```python
from build123d import *

# Parameters (mm, degrees)
F0_W     = 127
F0_H     = 127
F1_DEPTH = 127
F2_R     = 25.4
F3_R     = 12.7
F4_DEPTH = 50
F5_R     = 5
F6_DEPTH = 47
F7_R     = 5


# Not quite as in the source:
# - two fillets or chamfers of one size are made in one step


with BuildPart() as f1:
    # F0 (on Front) → F1 (new body)
    with BuildSketch(Plane.XZ):
        Rectangle(F0_W, F0_H)
    extrude(amount=F1_DEPTH)

    # F2
    f2_edges = [f1.edges().sort_by_distance(p)[0] for p in [
        (-63.5, -127, 0),
        (63.5, -127, 0),
        (-63.5, 0, 0),
        (63.5, 0, 0),
    ]]
    fillet(f2_edges, radius=F2_R)

    # F3
    f3_edges = [f1.edges().sort_by_distance(p)[0] for p in [
        (-63.5, -63.5, 63.5),
        (0, -127, -63.5),
        (63.5, -63.5, -63.5),
        (56.060512, -7.439488, -63.5),
        (56.060512, -119.560512, -63.5),
        (0, 0, -63.5),
        (-56.060512, -7.439488, -63.5),
        (-56.060512, -119.560512, -63.5),
        (-63.5, -63.5, -63.5),
    ]]
    fillet(f3_edges, radius=F3_R)

    # F4 (add): a face of the model
    f4_faces = [f1.faces().sort_by_distance(p)[0] for p in [
        (0, -63.5, 63.5),
    ]]
    extrude(f4_faces, amount=F4_DEPTH)

    # F5
    f5_edges = [f1.edges().sort_by_distance(p)[0] for p in [
        (-50.8, -63.5, 63.5),
        (-47.080256, -16.419744, 63.5),
        (-50.8, -63.5, 113.5),
        (-47.080256, -110.580256, 63.5),
        (0, -12.7, 63.5),
        (-47.080256, -16.419744, 113.5),
        (-47.080256, -110.580256, 113.5),
        (0, -12.7, 113.5),
        (0, -114.3, 113.5),
        (47.080256, -16.419744, 113.5),
        (47.080256, -110.580256, 113.5),
        (50.8, -63.5, 113.5),
        (0, -114.3, 63.5),
        (47.080256, -16.419744, 63.5),
        (47.080256, -110.580256, 63.5),
        (50.8, -63.5, 63.5),
    ]]
    fillet(f5_edges, radius=F5_R)

    # F6 (add): a face of the model
    f6_faces = [f1.faces().sort_by_distance(p)[0] for p in [
        (0, -63.5, 113.5),
    ]]
    extrude(f6_faces, amount=F6_DEPTH)

    # F7
    f7_edges = [f1.edges().sort_by_distance(p)[0] for p in [
        (-45.8, -63.5, 113.5),
        (-43.544722, -19.955278, 113.5),
        (-45.8, -63.5, 160.5),
        (-43.544722, -107.044722, 113.5),
        (0, -17.7, 113.5),
        (-43.544722, -19.955278, 160.5),
        (-43.544722, -107.044722, 160.5),
        (0, -17.7, 160.5),
        (0, -109.3, 160.5),
        (43.544722, -19.955278, 160.5),
        (43.544722, -107.044722, 160.5),
        (45.8, -63.5, 160.5),
        (0, -109.3, 113.5),
        (43.544722, -19.955278, 113.5),
        (43.544722, -107.044722, 113.5),
        (45.8, -63.5, 113.5),
    ]]
    fillet(f7_edges, radius=F7_R)


solid = f1.part
```
Input: part model. Units: mm. Frame: model coordinates. A direction names the side the tool comes from. Coordinates: 2 decimals unless noted, no trailing zeros. Loops run counter-clockwise (first coordinate to the right, second up) from the corner with the lowest first, then second, coordinate; pieces in that order, holes last. Notation, with made-up numbers: M 67.5,77.25 L 101.5,77.25 A12 cw 101.5,93.25 Z; hole C 35.25,49.5 d7. An arc over 180 degrees is marked long. Use a Markdown table: item, result. Add a question column.
1) Line query: L1, parallel to Y at x = -23.5, z = 149; L2, parallel to X at y = -48, z = 141.5; L3, parallel to Y at x = -1.5, z = 70. Output: solid intervals per line, ascending. Write a range as from..to.
2) Section C-C, the plane x = 19.5. Return the cut outline in (y, z).
3) Pin query (flat end, axial travel): P1, Ø19, axis at y = -57, z = 128, coming from the -X side; P2, Ø20.5, axis at y = -47, z = 88.5, coming from the +X side; P3, Ø2, axis at x = -4, y = -17.5, coming from the +Z side. Return the tip coordinate at first contact, or that it passes through.
4) Set-up query: faces 4 (the flat face through (50.8, -64, 88)), 5 (the cylindrical face through (46.98, -110.68, 87.85)), 6 (the flat face through (-1, -109.3, 136)), 7 (the cylindrical face through (-46.98, -16.32, 87.85)). Return all of +Z, -Z, +X, -X, +Y, -Y with unobstructed straight access to the full face (end or side cutting, diameter ignored); none if empty.
5) Draft query along Z for faces 1 (the flat face through (1, -12.7, 88)), 2 (the flat face through (-1, -63, -63.5)), 3 (the cylindrical face through (0.53, -107.87, 159)). Return one class per face: +Z half, -Z half, draft (parallel to the pull), parting line (faces both ways), or undercut.
6) Section B-B, the plane y = -99. Return the cut outline in (x, z).
7) Section D-D, the plane z = -5. Return the cut outline in (x, y), plus the area to 3 significant figures.
8) Section A-A, the plane z = 98. Return the cut outline in (x, y), plus the area to 3 significant figures.
Answer below:
| question | item | result |
|---|---|---|
| 1 | L1 | -109.3..-17.7 |
| 1 | L2 | -45.8..45.8 |
| 1 | L3 | -114.3..-12.7 |
| 2 | outline | M -127,-50.8 A12.7 ccw -114.3,-63.5 L -12.7,-63.5 A12.7 ccw 0,-50.8 L 0,50.8 A12.7 ccw -9.11,62.98 A5 cw -12.7,67.78 L -12.7,108.5 A5 ccw -15.2,112.83 A5 cw -17.7,117.16 L -17.7,155.5 A5 ccw -22.7,160.5 L -104.3,160.5 A5 ccw -109.3,155.5 L -109.3,117.16 A5 cw -111.8,112.83 A5 ccw -114.3,108.5 L -114.3,67.78 A5 cw -117.89,62.98 A12.7 ccw -127,50.8 Z |
| 3 | P1 | x = -45.8 |
| 3 | P2 | x = 50.8 |
| 3 | P3 | z = 158.21 |
| 4 | face 4 | +Z, +X, +Y, -Y |
| 4 | face 5 | +Z, +X, -Y |
| 4 | face 6 | +Z, +X, -X, -Y |
| 4 | face 7 | +Z, -X, +Y |
| 5 | face 1 | draft |
| 5 | face 2 | -Z half |
| 5 | face 3 | +Z half |
| 6 | outline | M -63.5,-50.8 A12.7 ccw -50.8,-63.5 L 50.8,-63.5 A12.7 ccw 63.5,-50.8 L 63.5,50.8 A12.7 ccw 54.39,62.98 A5 cw 50.8,67.78 L 50.8,108.5 A5 ccw 48.3,112.83 A5 cw 45.8,117.16 L 45.8,155.5 A5 ccw 40.8,160.5 L -40.8,160.5 A5 ccw -45.8,155.5 L -45.8,117.16 A5 cw -48.3,112.83 A5 ccw -50.8,108.5 L -50.8,67.78 A5 cw -54.39,62.98 A12.7 ccw -63.5,50.8 Z |
| 7 | outline | M -63.5,-101.6 A25.4 ccw -38.1,-127 L 38.1,-127 A25.4 ccw 63.5,-101.6 L 63.5,-25.4 A25.4 ccw 38.1,0 L -38.1,0 A25.4 ccw -63.5,-25.4 Z |
| 7 | area | 15,600 mm2 |
| 8 | outline | M -50.8,-101.6 A12.7 ccw -38.1,-114.3 L 38.1,-114.3 A12.7 ccw 50.8,-101.6 L 50.8,-25.4 A12.7 ccw 38.1,-12.7 L -38.1,-12.7 A12.7 ccw -50.8,-25.4 Z |
| 8 | area | 10,200 mm2 |
